```python
from build123d import *

# Parameters (mm, degrees)
BOSS_EXTRUDE1_DEPTH = 400
CHAMFER1_SIZE       = 0.3
LPATTERN1_COUNT     = 16
LPATTERN1_PITCH     = 25


with BuildPart() as part:
    # Sketch1 → Boss-Extrude1 (new body)
    with BuildSketch(Plane.XY):
        with BuildLine():
            Line((-6, 4), (6, 4))
            Line((6, 4), (6, 2.75))
            Line((6, 2.75), (6, 2.559016994))
            ThreePointArc((6, 2.559016994), (5.706107374, 2.475528258), (5.5, 2.25))
            Line((5.5, 2.25), (5, 2.25))
            Line((5, 2.25), (5, 1.75))
            Line((5, 1.75), (5.5, 1.75))
            ThreePointArc((5.5, 1.75), (5.706107374, 1.524471742), (6, 1.440983006))
            Line((6, 1.440983006), (6, 1.25))
            Line((6, 1.25), (6, -4))
            Line((6, -4), (-6, -4))
            Line((-6, -4), (-6, 1.25))
            Line((-6, 1.25), (-6, 1.440983006))
            ThreePointArc((-6, 1.440983006), (-5.706107374, 1.524471742), (-5.5, 1.75))
            Line((-5.5, 1.75), (-5, 1.75))
            Line((-5, 1.75), (-5, 2.25))
            Line((-5, 2.25), (-5.5, 2.25))
            ThreePointArc((-5.5, 2.25), (-5.706107374, 2.475528258), (-6, 2.559016994))
            Line((-6, 2.559016994), (-6, 2.75))
            Line((-6, 2.75), (-6, 4))
        make_face()
    extrude(amount=BOSS_EXTRUDE1_DEPTH)

    # Chamfer1
    chamfer1_edges = [part.edges().sort_by_distance(p)[0] for p in [
        (-6, 4, 200),
        (6, 4, 200),
        (6, -4, 200),
        (-6, -4, 200),
    ]]
    chamfer(chamfer1_edges, length=CHAMFER1_SIZE)

    # Sketch3 → M3 六角承窩頭蓋螺釘的柱孔1 (revolve, cut)
    with BuildSketch(Plane(origin=(0, 4, 12.5), x_dir=(0, 0, 1), z_dir=(1, 0, 0))):
        Polygon((0, 0), (0, 8), (2, 8), (1.75, 7.75), (1.75, 4.5), (3, 4.5), (3, 0.5), (3.5, 0), align=None)
    hole_wizard_m3_1 = revolve(axis=Axis((0, 10.35, 12.5), (0, -1, 0)), mode=Mode.SUBTRACT)

    # LPattern1: M3 六角承窩頭蓋螺釘的柱孔1 ×16
    with Locations(*[(0, 0, i * LPATTERN1_PITCH) for i in range(1, LPATTERN1_COUNT)]):
        add(hole_wizard_m3_1, mode=Mode.SUBTRACT)


solid = part.part
```
Check sheet for the modelled part. Datum: model origin and axes. Units: mm. Give positions to 0.01 mm unless a question says otherwise; leave off trailing zeros. Write each loop counter-clockwise with the first axis right and the second up, starting at its lowest first coordinate (ties: lowest second). Pieces come first, ordered by that corner, then holes. Notation, with made-up numbers: (44.5, 70.25) -> (91.5, 70.25) arc R10 cw to (91.5, 83.25) -> close; hole circle Ø10 at (3.5, 63.25). An arc over 180 degrees is marked (long way). Use CSV: the item, a comma, the result in double quotes. Start each with the question number.
Q1. Cross-section at B-B on z = 276. Enter the section's corners in (x, y).
Q2. Cross-section at A-A on y = -1.75. Count the separate pieces of the cut face and the enclosed holes in it, and give its area (3 significant figures).
Q3. Scan lines: line 1 along Y through (x, z) = (-5.5, 378); line 2 along X through (y, z) = (2.35, 12.5); line 3 along X through (y, z) = (2.05, 137.5). Record each from-to range of solid material in increasing order.
Q4. Depth check by flat-ended pin: P1, Ø3, axis at x = -0.5, z = 363, coming from the +Y side. Enter the tip coordinate at first touch or a pass-through.
Working result:
1,outline,"(-6, -3.7) -> (-5.7, -4) -> (5.7, -4) -> (6, -3.7) -> (6, 1.44) arc R0.56 cw to (5.5, 1.75) -> (5, 1.75) -> (5, 2.25) -> (5.5, 2.25) arc R0.56 cw to (6, 2.56) -> (6, 3.7) -> (5.7, 4) -> (-5.7, 4) -> (-6, 3.7) -> (-6, 2.56) arc R0.56 cw to (-5.5, 2.25) -> (-5, 2.25) -> (-5, 1.75) -> (-5.5, 1.75) arc R0.56 cw to (-6, 1.44) -> close"
2,separate pieces,"1"
2,enclosed holes,"16"
2,area,"4,650 mm^2"
3,line 1,"y = -4 to 1.75, 2.25 to 4"
3,line 2,"x = -5.56 to -3, 3 to 5.56"
3,line 3,"x = -5 to -3, 3 to 5"
4,P1,"stops at y = -0.5"
